Geometry check sheet. Reference: the model listing, model coordinates, mm. Face numbers are marked on the shaded views. A direction names the side the tool comes from. Round coordinates to 2 decimals unless told otherwise and drop trailing zeros. Loops run counter-clockwise (first coordinate to the right, second up) from the corner with the lowest first, then second, coordinate; pieces in that order, holes last. Notation, with made-up numbers: M -4.5,38 L 7.5,38 A28 ccw 7.5,72 Z; hole C 70.25,-0.75 d5. An arc over 180 degrees is marked long. Answer in a Markdown table with one row per item. Add a question column.
```python
from build123d import *

# Parameters (mm, degrees)
SKETCH1_W           = 23
SKETCH1_H           = 140
BOSS_EXTRUDE1_DEPTH = 3
SKETCH4_W           = 3
SKETCH4_H           = 140
BOSS_EXTRUDE3_DEPTH = 6.5
SKETCH3_R           = 2.85
CUT_EXTRUDE5_DEPTH  = 8.5


with BuildPart() as part:
    # Sketch1 → Boss-Extrude1 (new body)
    with BuildSketch(Plane.XY):
        Rectangle(SKETCH1_W, SKETCH1_H)
    extrude(amount=-BOSS_EXTRUDE1_DEPTH)

    # Sketch4 → Boss-Extrude3 (add)
    with BuildSketch(Plane.XY):
        with Locations((-10, 0)):
            Rectangle(SKETCH4_W, SKETCH4_H)
    extrude(amount=BOSS_EXTRUDE3_DEPTH)

    # Sketch3 → Cut-Extrude5 (cut)
    with BuildSketch(Plane.XY):
        with Locations((1.5, 59)):
            Circle(SKETCH3_R)
        with Locations((1.5, 29)):
            Circle(SKETCH3_R)
        with Locations((1.5, 9)):
            Circle(SKETCH3_R)
        with Locations((1.5, -21)):
            Circle(SKETCH3_R)
    extrude(amount=-CUT_EXTRUDE5_DEPTH, mode=Mode.SUBTRACT)


solid = part.part
```
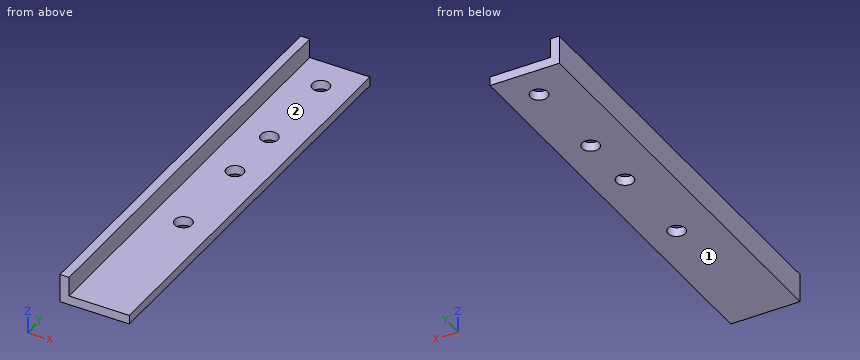
1) Cross-section at A-A, the plane x = 1.5. Record the boundary of the cut face in (y, z).
2) Cross-section at D-D, the plane x = 8.5. Record the boundary of the cut face in (y, z), plus the area to 3 significant figures.
3) Go/stop test with flat-tipped pins: pin 1 (2 mm diameter, centred on y = -12, z = 4.5, fed in from +X); pin 2 (7.5 mm diameter, centred on x = 1.5, y = 59, fed in from +Z). Record where each tip stops, or that it passes through.
4) Thickness scan on L1, parallel to Y at x = 1.5, z = -1.15; L2, parallel to X at y = -29.5, z = 4.5; L3, parallel to Z at x = 3.5, y = -11. Record the ranges inside material, lowest first. Write a range as [from, to].
5) Cross-section at C-C, the plane y = -49.5. Record the boundary of the cut face in (x, z), plus the area to 3 significant figures.
6) Set-up check for the marked faces 1 and 2: record each of +Z, -Z, +X, -X, +Y, -Y from which the full face is reachable in a straight line by a thin tool's end or side.
7) Cross-section at B-B, the plane y = -21. Record the boundary of the cut face in (x, z).
Worked answers:
| question | item | result |
|---|---|---|
| 1 | outline | M -70,-3 L -23.85,-3 L -23.85,0 L -70,0 Z; M -18.15,-3 L 6.15,-3 L 6.15,0 L -18.15,0 Z; M 11.85,-3 L 26.15,-3 L 26.15,0 L 11.85,0 Z; M 31.85,-3 L 56.15,-3 L 56.15,0 L 31.85,0 Z; M 61.85,-3 L 70,-3 L 70,0 L 61.85,0 Z |
| 2 | outline | M -70,-3 L 70,-3 L 70,0 L -70,0 Z |
| 2 | area | 420 mm2 |
| 3 | pin 1 | stops at x = -8.5 |
| 3 | pin 2 | stops at z = 0 |
| 4 | L1 | y = [-70, -23.85], [-18.15, 6.15], [11.85, 26.15], [31.85, 56.15], [61.85, 70] |
| 4 | L2 | x = [-11.5, -8.5] |
| 4 | L3 | z = [-3, 0] |
| 5 | outline | M -11.5,-3 L 11.5,-3 L 11.5,0 L -8.5,0 L -8.5,6.5 L -11.5,6.5 Z |
| 5 | area | 88.5 mm2 |
| 6 | face 1 | -Z, +X, -X, +Y, -Y |
| 6 | face 2 | +Z, +X, +Y, -Y |
| 7 | outline | M -11.5,-3 L -1.35,-3 L -1.35,0 L -8.5,0 L -8.5,6.5 L -11.5,6.5 Z; M 4.35,-3 L 11.5,-3 L 11.5,0 L 4.35,0 Z |
